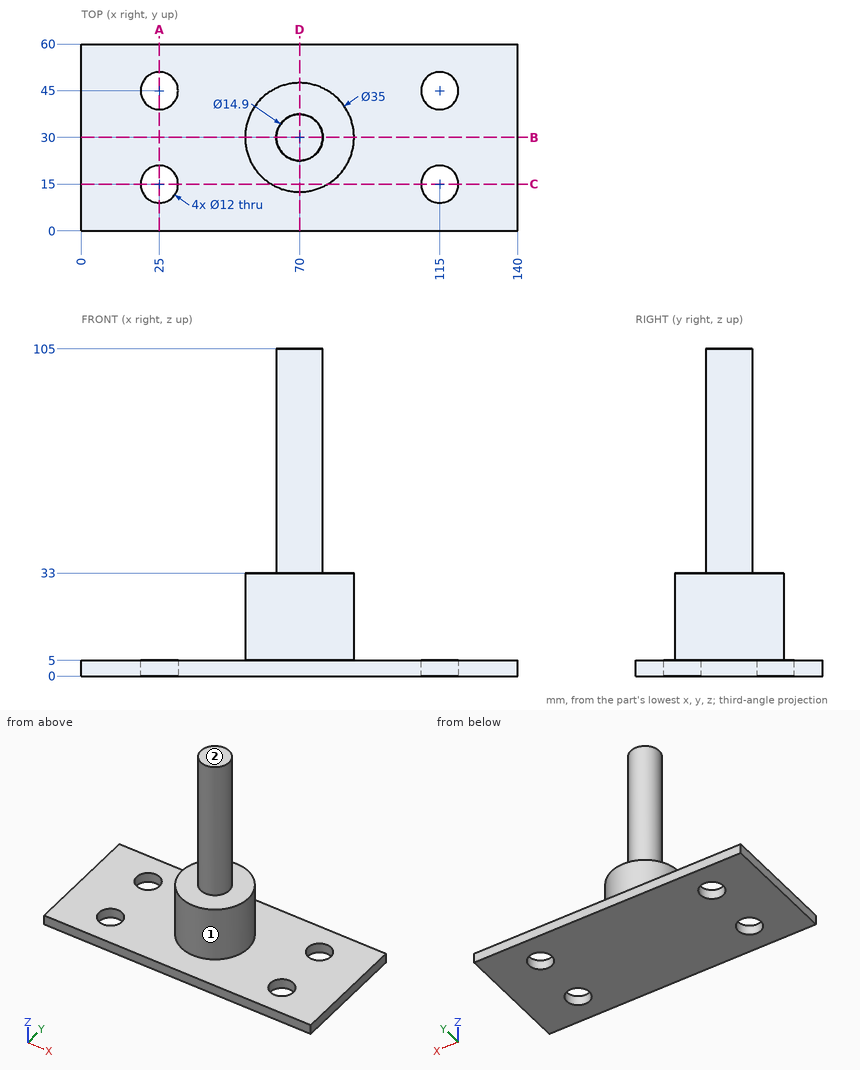
For this review, use the dimensioned drawing (mm, ordinates from the lowest corner) and the shaded views. A direction names the side the tool comes from. Give positions to 0.01 mm unless a question says otherwise; leave off trailing zeros. Loops run counter-clockwise (first coordinate to the right, second up) from the corner with the lowest first, then second, coordinate; pieces in that order, holes last.
Item 1: Take a section at D-D, the plane x = 70. State the section outline as (y, z) points, and give its area (3 significant figures).
Item 2: Take a section at C-C, the plane y = 15. State the section outline as (x, z) points, and give its area (3 significant figures).
Item 3: For line 1 along Y through (x, z) = (115, 3.5); line 2 along Z through (x, y) = (14.5, 21); line 3 along Z through (x, y) = (62, 33), list the stretches that pass through material, from the lowest coordinate up.
Item 4: Take a section at A-A, the plane x = 25. State the section outline as (y, z) points, and give its area (3 significant figures).
Item 5: Tool access review of the marked faces 1 and 2: name each direction out of +Z, -Z, +X, -X, +Y, -Y from which nothing blocks a thin tool from reaching the whole face with its end or side.
Item 6: Insertion check: pin 1 (6 mm diameter, centred on y = 23.5, z = 93, fed in from -X); pin 2 (6 mm diameter, centred on y = 20, z = 31.5, fed in from +X); pin 3 (12 mm diameter, centred on x = 78, z = 51.5, fed in from +Y). Each pin has a flat end and moves straight along its axis. Give the tip position at first contact, or say it passes through.
Item 7: Take a section at B-B, the plane y = 30. State the section outline as (x, z) points, and give its area (3 significant figures).
Calculated:
1. outline: (0, 0) - (60, 0) - (60, 5) - (47.5, 5) - (47.5, 33) - (37.45, 33) - (37.45, 105) - (22.55, 105) - (22.55, 33) - (12.5, 33) - (12.5, 5) - (0, 5) - close
1. area: 2,350 mm2
2. outline: (0, 0) - (19, 0) - (19, 5) - (0, 5) - close; (31, 0) - (109, 0) - (109, 5) - (79.01, 5) - (79.01, 33) - (60.99, 33) - (60.99, 5) - (31, 5) - close; (121, 0) - (140, 0) - (140, 5) - (121, 5) - close
2. area: 1,080 mm2
3. line 1: y = 0 to 9, 21 to 39, 51 to 60
3. line 2: z = 0 to 5
3. line 3: z = 0 to 33
4. outline: (0, 0) - (9, 0) - (9, 5) - (0, 5) - close; (21, 0) - (39, 0) - (39, 5) - (21, 5) - close; (51, 0) - (60, 0) - (60, 5) - (51, 5) - close
4. area: 180 mm2
5. face 1: +Z
5. face 2: +Z, +X, -X, +Y, -Y
6. pin 1: stops at x = 63.42
6. pin 2: stops at x = 86.04
6. pin 3: stops at y = 37.18
7. outline: (0, 0) - (140, 0) - (140, 5) - (87.5, 5) - (87.5, 33) - (77.45, 33) - (77.45, 105) - (62.55, 105) - (62.55, 33) - (52.5, 33) - (52.5, 5) - (0, 5) - close
7. area: 2,750 mm2
